Verification items for the finished model (mm, model axes). Round coordinates to 2 decimals unless told otherwise and drop trailing zeros. Order: outer loops, then holes, each group sorted by start corner. A loop starts at its lowest first (then second) coordinate and runs counter-clockwise, first axis right, second up. Notation, with made-up numbers: M 23,82 L 76,82 A21 cw 76,114 Z; hole C 81.5,42 d9. An arc over 180 degrees is marked long. Write item = value, one per line. Start each with the question number.
from build123d import *

# Parameters (mm, degrees)
SKETCH1_W               = 50.8
SKETCH1_H               = 101.6
BOSS_EXTRUDE2_DEPTH     = 101.6
SKETCH4_R               = 10.668
CUT_EXTRUDE2_DEPTH      = 51.8
CUT_EXTRUDE2_DEPTH_BACK = 51.8


with BuildPart() as part:
    # Sketch1 → Boss-Extrude2 (new body)
    with BuildSketch(Plane(origin=(0, 0, 0), x_dir=(1, 0, 0), z_dir=(0, 1, 0))):
        Rectangle(SKETCH1_W, SKETCH1_H)
    extrude(amount=BOSS_EXTRUDE2_DEPTH)

    # Sketch4 → Cut-Extrude2 (cut, two sides)
    with BuildSketch(Plane.XY) as cut_extrude2_sk:
        with Locations((0, 38.1)):
            Circle(SKETCH4_R)
    extrude(amount=CUT_EXTRUDE2_DEPTH, mode=Mode.SUBTRACT)
    extrude(cut_extrude2_sk.sketch, amount=-CUT_EXTRUDE2_DEPTH_BACK, mode=Mode.SUBTRACT)


solid = part.part
1) Scan lines: probe 1 along Y at (x, z) = (0.5, -22); probe 2 along X at (y, z) = (38.1, 15.5); probe 3 along Y at (x, z) = (-6, 0). Record each from-to range of solid material in increasing order.
2) Gauge pin test, flat end, axial feed: P1, Ø24.5, axis at x = 0, y = 38.1, coming from the -Z side. Record the tip position at first contact, or that the pin passes through.
3) Cross-section at B-B, the plane y = 38.1. Enter the section's corners in (x, z), then the cut area to 3 significant figures.
4) Cross-section at C-C, the plane z = 32.5. Enter the section's corners in (x, y), then the cut area to 3 significant figures.
5) Cross-section at A-A, the plane x = 0. Enter the section's corners in (y, z), then the cut area to 3 significant figures.
Geometry results:
q1.probe_1 = 0 to 27.44, 48.76 to 101.6
q1.probe_2 = -25.4 to -10.67, 10.67 to 25.4
q1.probe_3 = 0 to 29.28, 46.92 to 101.6
q2.P1 = -50.8
q3.outline = M -25.4,-50.8 L -10.67,-50.8 L -10.67,50.8 L -25.4,50.8 Z; M 10.67,-50.8 L 25.4,-50.8 L 25.4,50.8 L 10.67,50.8 Z
q3.area = 2,990 mm^2
q4.outline = M -25.4,0 L 25.4,0 L 25.4,101.6 L -25.4,101.6 Z; hole C 0,38.1 d21.34
q4.area = 4,800 mm^2
q5.outline = M 0,-50.8 L 27.43,-50.8 L 27.43,50.8 L 0,50.8 Z; M 48.77,-50.8 L 101.6,-50.8 L 101.6,50.8 L 48.77,50.8 Z
q5.area = 8,150 mm^2
